```python
from build123d import *

# Parameters (mm, degrees)
EXTRUDE_DEPTH = 110
POCKET_DEPTH  = 5
FILLET_R      = 1
FILLET001_R   = 0.5
SKETCH002_R   = 3
PAD_DEPTH     = 3


with BuildPart() as part:
    # Sketch → Extrude (new body)
    with BuildSketch(Plane.XY):
        Polygon((0, 0), (12, 0), (12, 8), (10, 8), (10, 2), (2, 2), (2, 8), (0, 8), align=None)
    extrude(amount=EXTRUDE_DEPTH)

    # Sketch001 (on Face5 of BaseFeature) → Pocket (cut)
    with BuildSketch(Plane(origin=(0, 2, 0), x_dir=(-1, 0, 0), z_dir=(0, 1, 0))):
        with BuildLine():
            ThreePointArc((-4.5, 105), (-6, 106.5), (-7.5, 105))
            Line((-7.5, 105), (-7.5, 5))
            ThreePointArc((-7.5, 5), (-6, 3.5), (-4.5, 5))
            Line((-4.5, 105), (-4.5, 5))
        make_face()
    extrude(amount=-POCKET_DEPTH, mode=Mode.SUBTRACT)

    # Fillet
    fillet_edges = [part.edges().sort_by_distance(p)[0] for p in [
        (11, 8, 0),
        (10, 5, 0),
        (2, 5, 0),
        (1, 8, 0),
        (11, 8, 110),
        (10, 5, 110),
        (2, 5, 110),
        (1, 8, 110),
    ]]
    fillet(fillet_edges, radius=FILLET_R)

    # Fillet001
    fillet001_edges = [part.edges().sort_by_distance(p)[0] for p in [
        (0, 3.5, 0),
        (12, 3.5, 0),
    ]]
    fillet(fillet001_edges, radius=FILLET001_R)

    # Sketch002 (on Face2 of Fillet001) → Pad (join)
    with BuildSketch(Plane.XZ):
        with BuildLine():
            Line((0, 0.5), (0, -19.5))
            ThreePointArc((0, -19.5), (6, -25.5), (12, -19.5))
            Line((12, -19.5), (12, 0.5))
            Line((12, 0.5), (0, 0.5))
        make_face()
        with Locations((6, -19.5)):
            Circle(SKETCH002_R, mode=Mode.SUBTRACT)
    extrude(amount=-PAD_DEPTH)


solid = part.part
```
For this review, take the finished solid that the model builds, in its own axes (mm). A direction names the side the tool comes from. Coordinates: 2 decimals unless noted, no trailing zeros. Loops run counter-clockwise (first coordinate to the right, second up) from the corner with the lowest first, then second, coordinate; pieces in that order, holes last.
1. Add section A-A, the plane z = 10. Give the boundary of the cut face in (x, y), then the cut area to 3 significant figures.
2. For faces 5 (the flat face through (4, 2, 54)), 6 (the flat face through (0, 4, 46)), list the 3-axis set-ups (+Z, -Z, +X, -X, +Y, -Y) from which the entire face can be reached by the end or side of a thin tool; tool diameter is ignored.
3. Add section B-B, the plane x = 6. Give the boundary of the cut face in (y, z).
4. Insertion check: P1, Ø1.5, axis at x = 3, z = 29.5, coming from the +Y side; P2, Ø0.5, axis at x = 5.5, y = 2.5, coming from the +Z side; P3, Ø5, axis at x = 8, z = -10.5, coming from the +Y side. Each pin has a flat end and moves straight along its axis. Give the tip position at first contact, or say it passes through.
5. For line 1 (Z direction, x = 6, y = 1.6); line 2 (Z direction, x = 6, y = 2.25); line 3 (X direction, y = 2.5, z = 19), list the stretches that pass through material, from the lowest coordinate up.
6. Mouldability with a two-part tool opening along Z and no side actions: class faces 1 (the cylindrical face through (5.9, 1.5, -25.5)), 2 (the flat face through (10, 5, 54)), 3 (the flat face through (6, 1, 110)), 4 (the cylindrical face through (5.35, 1.48, -22.43)) as +Z half, -Z half, draft (parallel to the pull), parting line (faces both ways), or undercut.
Result:
1. outline: (0, 0) - (4.5, 0) - (4.5, 2) - (2, 2) - (2, 8) - (0.5, 8) arc R0.5 ccw to (0, 7.5) - close; (7.5, 0) - (12, 0) - (12, 7.5) arc R0.5 ccw to (11.5, 8) - (10, 8) - (10, 2) - (7.5, 2) - close
1. area: 41.9 mm2
2. face 5: +Z, +Y
2. face 6: +Z, -Z, -X, +Y, -Y
3. outline: (0, -25.5) - (3, -25.5) - (3, -22.5) - (0, -22.5) - close; (0, -16.5) - (3, -16.5) - (3, 0.5) - (2, 0.5) - (2, 3.5) - (0, 3.5) - close; (0, 106.5) - (2, 106.5) - (2, 110) - (0, 110) - close
4. P1: stops at y = 2
4. P2: stops at z = 0.5
4. P3: stops at y = 3
5. line 1: z = -25.5 to -22.5, -16.5 to 3.5, 106.5 to 110
5. line 2: z = -25.5 to -22.5, -16.5 to 0.5
5. line 3: x = 0 to 2, 10 to 12
6. face 1: -Z half
6. face 2: draft
6. face 3: +Z half
6. face 4: undercut
